Print and shaded views of the part. All mm, measured from the part's lowest x, y and z. Give positions to 0.01 mm unless a question says otherwise; leave off trailing zeros. Loops run counter-clockwise (first coordinate to the right, second up) from the corner with the lowest first, then second, coordinate; pieces in that order, holes last. Notation, with made-up numbers: M -36,7 L -9,7 A28 ccw -9,37 Z; hole C 45,-12.75 d6. An arc over 180 degrees is marked long. Answer as CSV lines item,"result".
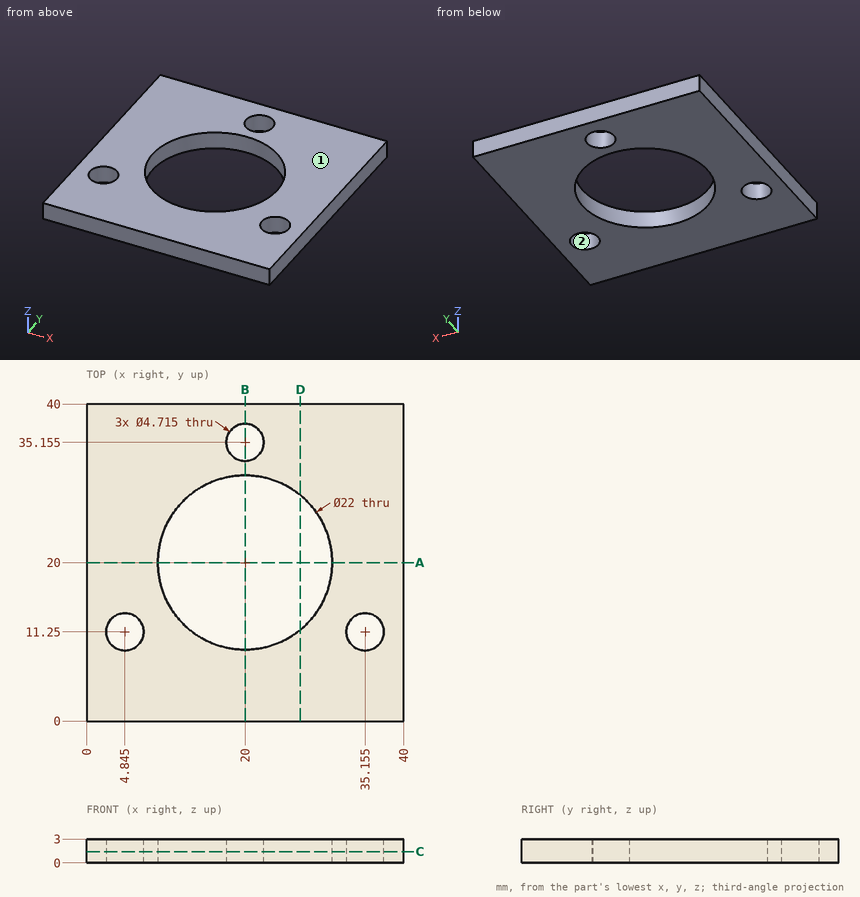
Q1. Pin check, flat tip, straight feed: P1, Ø7.5, axis at x = 35.16, y = 11.25, coming from the +Z side. Stop position of the tip, or through.
Solution:
P1,"stops at z = 3"
Q2. Cut at C-C (z = 1.4). Give the number of separate pieces and of enclosed holes in the cut face, and give its area (3 significant figures).
Solution:
separate pieces,"1"
enclosed holes,"4"
area,"1,170 mm²"
Q3. Wall check: line 1 (Y direction, x = 20, z = 1.6); line 2 (X direction, y = 20, z = 0.6); line 3 (X direction, y = 10, z = 2.75) (1 decimal). Give the ranges that are in metal, low to high. Write a range as [from, to].
Solution:
line 1,"y = [0, 9], [31, 32.8], [37.51, 40]"
line 2,"x = [0, 9], [31, 40]"
line 3,"x = [0, 2.8], [6.8, 15.4], [24.6, 33.2], [37.2, 40]"
Q4. Cut at D-D (x = 27). Write the cut outline in (y, z) (1 decimal).
Solution:
outline,"M 0,0 L 11.5,0 L 11.5,3 L 0,3 Z; M 28.5,0 L 40,0 L 40,3 L 28.5,3 Z"
Q5. Cut at A-A (y = 20). Write the cut outline in (x, z).
Solution:
outline,"M 0,0 L 9,0 L 9,3 L 0,3 Z; M 31,0 L 40,0 L 40,3 L 31,3 Z"
Q6. Mould opens along Y. For the marked faces 1 and 2 say: released by +Y, released by -Y, zero draft, split by the parting line, or undercut.
Solution:
face 1,"zero draft"
face 2,"undercut"
Q7. Cut at B-B (x = 20). Write the cut outline in (y, z).
Solution:
outline,"M 0,0 L 9,0 L 9,3 L 0,3 Z; M 31,0 L 32.8,0 L 32.8,3 L 31,3 Z; M 37.51,0 L 40,0 L 40,3 L 37.51,3 Z"
